Could you check a few things on this model? Use its own coordinates, in mm. A direction names the side the tool comes from. Round coordinates to 2 decimals unless told otherwise and drop trailing zeros. Write each loop counter-clockwise with the first axis right and the second up, starting at its lowest first coordinate (ties: lowest second). Pieces come first, ordered by that corner, then holes. Notation, with made-up numbers: (-23, -30.75) -> (34, -30.75) arc R24 ccw to (34, -17.75) -> close; hole circle Ø6 at (43.25, 52). An arc over 180 degrees is marked (long way). Return JSON: item names as keys, results as strings.
Autodesk Inventor part; units mm, degrees
ref_plane "YZ Plane" through (0, 0, 0) normal (1, 0, 0) x (0, 1, 0)
ref_plane "XZ Plane" through (0, 0, 0) normal (0, 1, 0) x (-1, 0, 0)
ref_plane "XY Plane" through (0, 0, 0) normal (0, 0, 1) x (1, 0, 0)
sketch "Sketch1" plane through (0, 0, 0) normal (0, 1, 0) x (-1, 0, 0)
  circle A0 centre (0, 0) radius 48
  circle A1 centre (0, 0) radius 45
  line L0 (10, -45) -> (-10, -45)
  line L1 (-10, -45) -> (-10, -80)
  line L2 (-10, -80) -> (10, -80)
  line L3 (10, -80) -> (10, -45)
  line L4 (-4, 44.8219) -> (4, 44.8219)
  circle A2 centre (0, -70) radius 10
  circle A3 centre (0, -70) radius 2
  line L5 (0, 0) -> (-57.7849, -57.7849)
  line L6 (0, 0) -> (0, -45)
  line L7 (-26.4827, -36.3822) -> (-36.3822, -26.4827)
  line L8 (-36.3822, -26.4827) -> (-46.9888, -37.0893)
  line L9 (-46.9888, -37.0893) -> (-37.0893, -46.9888)
  line L10 (-37.0893, -46.9888) -> (-26.4827, -36.3822)
  line L11 (-29.3111, -33.5538) -> (-33.5538, -29.3111)
  line L12 (-33.5538, -29.3111) -> (-44.1604, -39.9177)
  line L13 (-44.1604, -39.9177) -> (-39.9177, -44.1604)
  line L14 (-39.9177, -44.1604) -> (-29.3111, -33.5538)
  point P0 (0, 45)
  point P1 (4, 60)
  point P2 (-10, -46.9468)
  point P3 (10, -46.9468)
  point P4 (10, -70)
  point P5 (-10, -70)
  point P6 (0, -45)
  point P7 (0, -80)
  point P8 (-28.6285, -38.528)
  point P9 (-38.528, -28.6285)
  point P10 (-29.6277, -33.8703)
  point P11 (-33.8703, -29.6277)
  dimension "d0" = 96
  dimension "d1" = 90
  dimension "d2" = 20
  dimension "d13" = 35
  dimension "d14" = 4
  dimension "d15" = 45
  dimension "d16" = 7
  dimension "d17" = 7
  dimension "d18" = 15
  dimension "d19" = 3
  dimension "d20" = 3
extrude "Extrusion1" add sketch "Sketch1" along normal blind 15 contours A0 L3 L0 A1 L8 | L8 A1 L12 A0 | A0 L12 L9 L8 | L3 A2 L1 A0 | A0 L1 L0 L3 | A0 L10 A1 L0 L1 | A2 | L3 L2 A2 | L10 L9 L14 A0 | A0 L14 A1 L10 | A2 L2 L1
fillet "Fillet1" radius 5 6 edges at (38.528, 7.5, -28.6285) (28.6285, 7.5, -38.528) (10, 7.5, -46.9468) (-10, 7.5, -46.9468) (33.8703, 7.5, -29.6277) (29.6277, 7.5, -33.8703)
sketch "Sketch5" plane through (10, 0, -80) normal (1, 0, 0) x (0, 0, -1)
  line L0 (0, 15) -> (-29.1669, 15)
  line L1 (0, 0) -> (0, 15)
  line L2 (-29.1669, 15) -> (0, 15)
  line L3 (0, 15) -> (0, 7.5)
  line L4 (0, 7.5) -> (-29.1669, 7.5)
  line L5 (-29.1669, 7.5) -> (-29.1669, 15)
  arc A0 (-29.1669, 15) -> (-21.6669, 7.5) centre (-21.6669, 15) ccw
  line L6 (-29.1669, 0) -> (-29.1669, 15)
  point P0 (-80, 0)
extrude "Extrusion3" cut sketch "Sketch5" against normal through all contours L1 L4 A0 L0
fillet "Fillet2" radius 7 2 edges at (10, 3.75, -80) (-10, 3.75, -80)
sketch "Sketch6" plane through (46.9888, 0, -37.0893) normal (0.7071, 0, 0.7071) x (0.7071, 0, -0.7071)
  circle A0 centre (-3.9143, 7.5) radius 2
  line L0 (0, 0) -> (0, 15)
  line L1 (-7.8286, 15) -> (0, 15)
  point P0 (-59.4522, 0)
  point P1 (0, 7.5)
  point P2 (-3.9143, 15)
  dimension "d25" = 4
extrude "Extrusion4" cut sketch "Sketch6" against normal up to surface (14 mm away)
fillet "Fillet3" radius 2 1 edges at (0, 15, -50.8331)
fillet "Fillet4" radius 2 5 edges at (-31.8198, 15, 31.8198) (29.6443, 15, -35.5728) (36.3481, 15, -40.5908) (35.5728, 15, -29.6443) (40.5908, 15, -36.3481)
properties part number "HopperMount"
1) I want a section at D-D, the plane y = 11.25. Please give me the cut outline in (x, z), and give its area (3 significant figures).
Return value:
{"outline": "(-13.58, -46.04) arc R5 cw to (-10, -50.83) -> (-10, -51.84) -> (10, -51.84) -> (10, -50.83) arc R5 cw to (13.58, -46.04) arc R48 ccw to (25.37, -40.74) arc R5 cw to (31.55, -41.45) -> (37.09, -46.99) -> (39.92, -44.16) -> (32.78, -37.02) arc R5 ccw to (26.32, -36.5) arc R45 cw (long way) to (36.5, -26.32) arc R5 ccw to (37.02, -32.78) -> (44.16, -39.92) -> (46.99, -37.09) -> (41.45, -31.55) arc R5 cw to (40.74, -25.37) arc R48 ccw (long way) to start", "area": "1,040 mm²"}
2) For faces 4 (the face through (35.6, 9.1, -45.5)), 5 (the face through (43, 9.1, -33.1)), 6 (the face through (39.748, 6.409, -35.505)), 7 (the face through (35.973, 14.43, -41.066)), which set-ups out of +Z, -Z, +X, -X, +Y, -Y let a thin tool reach every point of the face, with its end or its side?
Return value:
{"face 4": "-Z, +Y, -Y", "face 5": "+X, +Y, -Y", "face 6": "+Y, -Y", "face 7": "+Y"}
3) I want a section at C-C, the plane y = 1.75. Please give me the cut outline in (x, z).
Return value:
{"outline": "(-13.58, -46.04) arc R5 cw to (-10, -50.83) -> (-10, -73) arc R7 ccw to (-3, -80) -> (3, -80) arc R7 ccw to (10, -73) -> (10, -50.83) arc R5 cw to (13.58, -46.04) arc R48 ccw to (25.37, -40.74) arc R5 cw to (31.55, -41.45) -> (37.09, -46.99) -> (39.92, -44.16) -> (32.78, -37.02) arc R5 ccw to (26.32, -36.5) arc R45 cw (long way) to (36.5, -26.32) arc R5 ccw to (37.02, -32.78) -> (44.16, -39.92) -> (46.99, -37.09) -> (41.45, -31.55) arc R5 cw to (40.74, -25.37) arc R48 ccw (long way) to start; hole circle Ø4 at (0, -70)"}
4) Thinking about a two-plate mould opening in Z: for faces 1 (the face through (19.576, 7.395, -43.827)), 2 (the face through (40.966, 14.43, -35.873)), 3 (the face through (25, 15, -40)), which applies, pulls with the +Z half, pulls with the -Z half, needs draft (parallel to the pull), parting line crosses it, or undercut?
Return value:
{"face 1": "pulls with the -Z half", "face 2": "undercut", "face 3": "needs draft"}
5) I want a section at B-B, the plane z = 0. Please give me the cut outline in (x, y).
Return value:
{"outline": "(-48, 0) -> (-45, 0) -> (-45, 13) arc R2 ccw to (-47, 15) -> (-48, 15) -> close; (45, 0) -> (48, 0) -> (48, 15) -> (47, 15) arc R2 ccw to (45, 13) -> close"}
6) Will these pins go through, and if not, where does the flat tip stop? pin 1 Ø22 at (x, z) = (2.5, -69.5) entering from +Y; pin 2 Ø6 at (y, z) = (5, -23) entering from +X; pin 3 Ø4 at (y, z) = (2.5, -64.5) entering from +X.
Return value:
{"pin 1": "y = 7.5", "pin 2": "x = 43.63", "pin 3": "x = 10"}
7) I want a section at A-A, the plane x = 0. Please give me the cut outline in (y, z), and give its area (3 significant figures).
Return value:
{"outline": "(0, -80) -> (7.5, -80) -> (7.5, -72) -> (0, -72) -> close; (0, -68) -> (7.5, -68) -> (7.5, -58.33) arc R7.5 cw to (13.42, -51) arc R2 ccw to (15, -49.05) -> (15, -47) arc R2 ccw to (13, -45) -> (0, -45) -> close; (0, 45) -> (13, 45) arc R2 ccw to (15, 47) -> (15, 48) -> (0, 48) -> close", "area": "331 mm²"}
8) If I drill on probe 1 along Z at (x, y) = (0, 3); probe 2 along X at (y, z) = (4.5, 0); probe 3 along X at (y, z) = (2, -36), over which ranges is the centre line in solid material (lowest first)? Write a range as [from, to].
Return value:
{"probe 1": "[-80, -72], [-68, -45], [45, 48]", "probe 2": "[-48, -45], [45, 48]", "probe 3": "[-31.75, -27], [27.18, 31.3], [40.24, 45.9]"}
